Build history of the part. All positions in model axes, mm. Face numbers are marked on the shaded views. A direction names the side the tool comes from. Round coordinates to 2 decimals unless told otherwise and drop trailing zeros. Order: outer loops, then holes, each group sorted by start corner. A loop starts at its lowest first (then second) coordinate and runs counter-clockwise, first axis right, second up. Notation, with made-up numbers: (37.25, -38.5) -> (53.25, -38.5) arc R28 cw to (53.25, -10.5) -> close; hole circle Ø11 at (62, 61). An arc over 180 degrees is marked (long way). Use a Markdown table: item, result. Add a question column.
Item 1: 3-axis set-ups, long thin cutter, end or side, ignore diameter. For the marked faces 1 and 2: which of +Z, -Z, +X, -X, +Y, -Y reach the whole face in a straight line?
Item 2: Slice it at A-A, the plane x = 0. Give the cut face in (y, z), plus the area to 3 significant figures.
Item 3: Pin check, flat tips, straight feed: pin 1 (5 mm diameter, centred on x = 1.5, z = 6, fed in from +Y); pin 2 (4 mm diameter, centred on x = -3.5, z = 3, fed in from -Y); pin 3 (1 mm diameter, centred on x = 1.5, z = 7.5, fed in from -Y); pin 4 (1.6 mm diameter, centred on x = -1, y = 0, fed in from +Z). Stop position of each tip, or through.
Item 4: Probe L1, parallel to Y at x = 0, z = 9.5; L2, parallel to Y at x = 1.75, z = 10.25; L3, parallel to X at y = -1.5, z = 11. List the from-to ranges inside material, lowest first.
Item 5: Two-plate mould, pull along X, no slides. Class the marked faces 3, 4 and 5: released by +X, released by -X, zero draft, split by the parting line, or undercut.
Item 6: Slice it at B-B, the plane z = 10.5. Give the cut face in (x, y), plus the area to 3 significant figures.
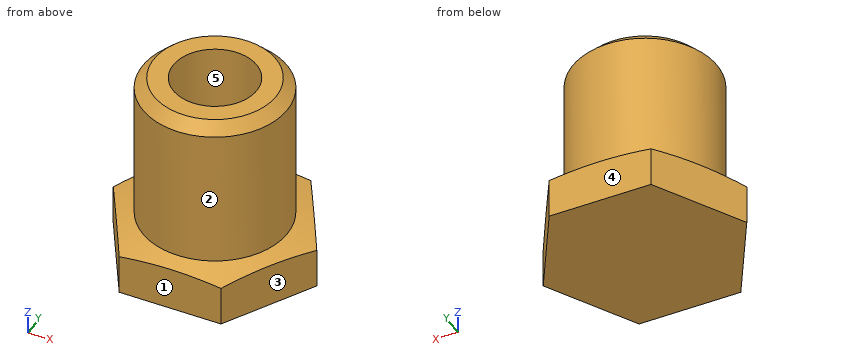
from build123d import *

# Parameters (mm, degrees)
BOSS_EXTRUDE1_DEPTH = 3
SKETCH2_R           = 4.5
BOSS_EXTRUDE2_DEPTH = 9.4
CUT_EXTRUDE1_START  = -2
SKETCH3_R           = 2.6
CUT_EXTRUDE1_DEPTH  = 13.978095117
CHAMFER2_SIZE       = 0.7


with BuildPart() as part:
    # Sketch1 → Boss-Extrude1 (new body)
    with BuildSketch(Plane.XY):
        Polygon((6.350852961, 0), (3.175426481, 5.5), (-3.175426481, 5.5), (-6.350852961, 0), (-3.175426481, -5.5), (3.175426481, -5.5), align=None)
    extrude(amount=BOSS_EXTRUDE1_DEPTH)

    # Sketch2 → Boss-Extrude2 (add)
    with BuildSketch(Plane.XY.offset(3)):
        Circle(SKETCH2_R)
    extrude(amount=BOSS_EXTRUDE2_DEPTH)

    # Sketch3 → Cut-Extrude1 (cut, through all)
    with BuildSketch(Plane(origin=(0, 0, 0), x_dir=(-1, 0, 0), z_dir=(0, 0, -1)).offset(CUT_EXTRUDE1_START)):
        Circle(SKETCH3_R)
    extrude(amount=-CUT_EXTRUDE1_DEPTH, mode=Mode.SUBTRACT)

    # Sketch5 → Cut-Revolve2 (revolve, cut)
    with BuildSketch(Plane(origin=(0, 0, 0), x_dir=(1, 0, 0), z_dir=(0, 1, 0)), mode=Mode.PRIVATE) as cut_revolve2_sk:
        Polygon((-4.5, -3), (-6.350852961, -3), (-6.350852961, -2.5), align=None)
    revolve(cut_revolve2_sk.sketch.rotate(Axis((0, 0, 12.4), (0, 0, -1)), 180), axis=Axis((0, 0, 12.4), (0, 0, -1)), mode=Mode.SUBTRACT)

    # Chamfer2
    chamfer2_edges = [part.edges().sort_by_distance(p)[0] for p in [
        (-4.5, 0, 12.4),
    ]]
    chamfer(chamfer2_edges, length=CHAMFER2_SIZE)


solid = part.part
Check sheet entries:
| question | item | result |
|---|---|---|
| 1 | face 1 | +Z, -Z, +X, -X, -Y |
| 1 | face 2 | +Z |
| 2 | outline | (-5.5, 0) -> (5.5, 0) -> (5.5, 2.73) -> (4.5, 3) -> (4.5, 11.7) -> (3.8, 12.4) -> (2.6, 12.4) -> (2.6, 2) -> (-2.6, 2) -> (-2.6, 12.4) -> (-3.8, 12.4) -> (-4.5, 11.7) -> (-4.5, 3) -> (-5.5, 2.73) -> close |
| 2 | area | 62.8 mm2 |
| 3 | pin 1 | y = 4.5 |
| 3 | pin 2 | y = -5.5 |
| 3 | pin 3 | y = -4.39 |
| 3 | pin 4 | z = 2 |
| 4 | L1 | -4.5 to -2.6, 2.6 to 4.5 |
| 4 | L2 | -4.15 to -1.92, 1.92 to 4.15 |
| 4 | L3 | -4.24 to -2.12, 2.12 to 4.24 |
| 5 | face 3 | released by +X |
| 5 | face 4 | zero draft |
| 5 | face 5 | undercut |
| 6 | outline | circle Ø9 at (0, 0); hole circle Ø5.2 at (0, 0) |
| 6 | area | 42.4 mm2 |
